For this review, use the dimensioned drawing (mm, ordinates from the lowest corner) and the shaded views. A direction names the side the tool comes from. Coordinates: 2 decimals unless noted, no trailing zeros. Loops run counter-clockwise (first coordinate to the right, second up) from the corner with the lowest first, then second, coordinate; pieces in that order, holes last. Notation, with made-up numbers: (-11.5, 24.25) - (20.5, 24.25) arc R21 ccw to (20.5, 37.25) - close; hole circle Ø4 at (-40, 87.5). An arc over 180 degrees is marked (long way). One line per item, written item: value. Start each with the question number.
1. We need section D-D, the plane x = 6. Give the boundary of the cut face in (y, z), then the cut area to 3 significant figures.
2. To check wall thickness, follow line 1 (X direction, y = 26, z = 43.5); line 2 (Y direction, x = 66, z = 4); line 3 (Z direction, x = 55, y = 29). State the ranges of each line that lie inside material, in increasing order.
3. For the marked faces 5 and 6, list the 3-axis set-ups (+Z, -Z, +X, -X, +Y, -Y) from which the entire face can be reached by the end or side of a thin tool; tool diameter is ignored.
4. Mouldability with a two-part tool opening along X and no side actions: class the marked faces 1, 2, 3 and 4 as +X half, -X half, draft (parallel to the pull), parting line (faces both ways), or undercut.
5. Insertion check: P1, Ø1.5, axis at y = 19.5, z = 23.5, coming from the -X side; P2, Ø8, axis at y = 13.5, z = 28.5, coming from the -X side; P3, Ø2, axis at x = 1, y = 27, coming from the +Z side; P4, Ø12, axis at x = 17, y = 21, coming from the +Z side. Each pin has a flat end and moves straight along its axis. Give the tip position at first contact, or say it passes through.
6. We need section C-C, the plane y = 24.5. Give the boundary of the cut face in (x, z).
7. We need section A-A, the plane z = 12.5. Give the boundary of the cut face in (x, y).
8. We need section B-B, the plane y = 11. Give the boundary of the cut face in (x, z).
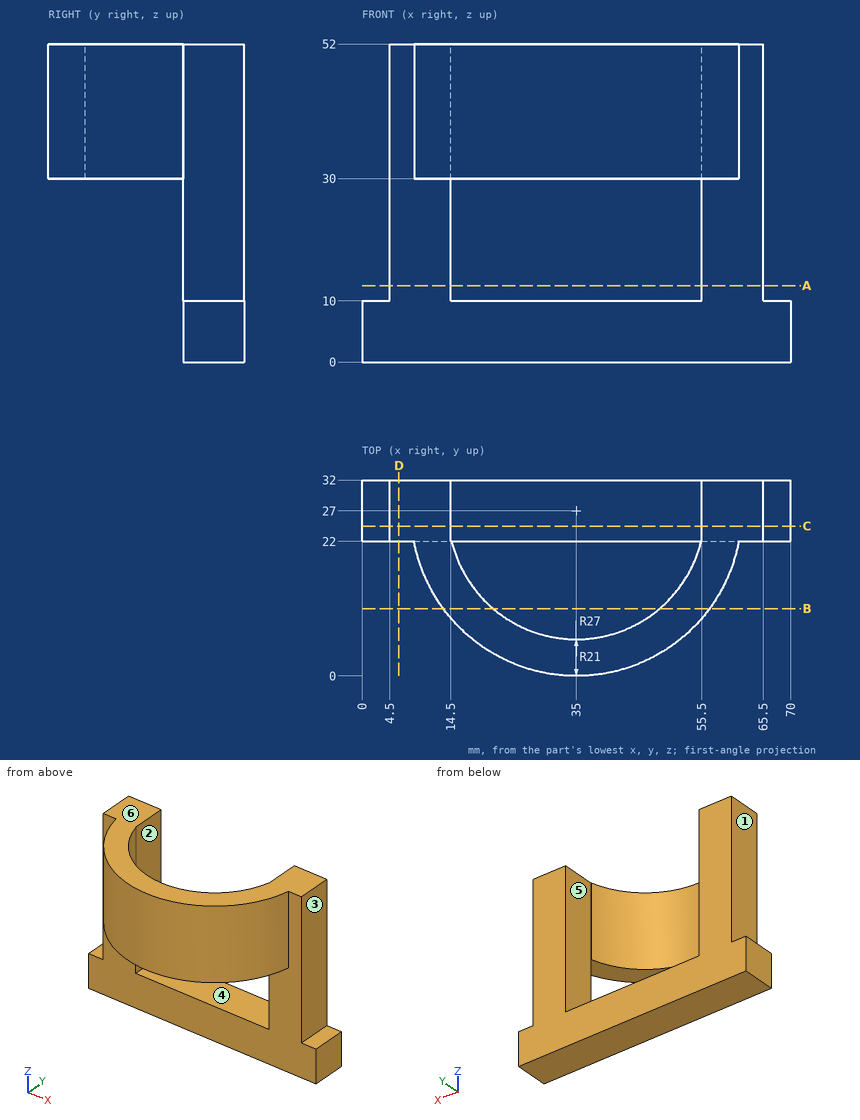
Findings below:
1. outline: (22, 0) - (32, 0) - (32, 52) - (22, 52) - close
1. area: 520 mm2
2. line 1: 4.5 to 14.5, 55.5 to 65.5
2. line 2: 22 to 32
2. line 3: 0 to 10
3. face 5: +Z, +Y
3. face 6: +Z, +X, -X, +Y, -Y
4. face 1: -X half
4. face 2: undercut
4. face 3: +X half
4. face 4: undercut
5. P1: through
5. P2: x = 9.84
5. P3: z = 10
5. P4: z = 52
6. outline: (0, 0) - (70, 0) - (70, 10) - (65.5, 10) - (65.5, 52) - (55.5, 52) - (55.5, 10) - (14.5, 10) - (14.5, 52) - (4.5, 52) - (4.5, 10) - (0, 10) - close
7. outline: (4.5, 22) - (14.5, 22) - (14.5, 32) - (4.5, 32) - close; (55.5, 22) - (65.5, 22) - (65.5, 32) - (55.5, 32) - close
8. outline: (13.25, 30) - (21.4, 30) - (21.4, 52) - (13.25, 52) - close; (48.6, 30) - (56.75, 30) - (56.75, 52) - (48.6, 52) - close
